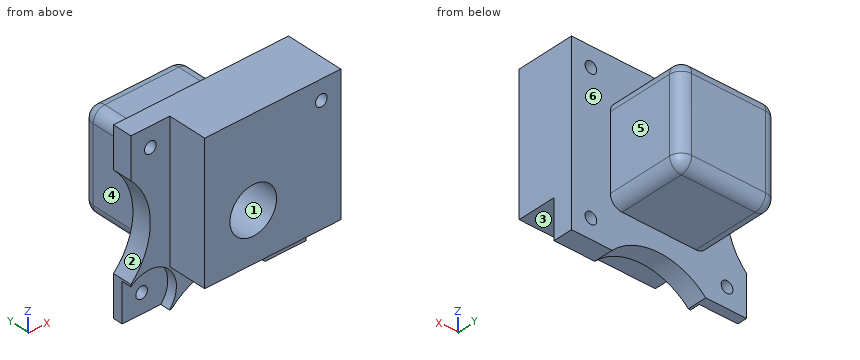
from build123d import *

# Parameters (mm, degrees)
SKETCH1_W               = 45
SKETCH1_H               = 45
BOSS_EXTRUDE1_DEPTH     = 15
CUT_EXTRUDE1_DEPTH      = 10
CUT_EXTRUDE2_DEPTH      = 38.243644172
CUT_EXTRUDE2_DEPTH_BACK = 38.243644172
CUT_EXTRUDE3_DEPTH      = 2.5
SKETCH5_W               = 25
SKETCH5_H               = 25
BOSS_EXTRUDE2_DEPTH     = 20
FILLET1_R               = 3
SKETCH6_R               = 6
CUT_EXTRUDE4_DEPTH      = 28.99918
SKETCH7_W               = 13
SKETCH7_H               = 13
CUT_EXTRUDE5_DEPTH      = 13
FILLET2_R               = 3
CUT_EXTRUDE6_DEPTH      = 42.074189356
CUT_EXTRUDE6_DEPTH_BACK = 42.074189356
SKETCH8_R               = 1.5


with BuildPart() as part:
    # Sketch1 → Boss-Extrude1 (new body)
    with BuildSketch(Plane(origin=(0, 0, 0), x_dir=(1, 0, 0), z_dir=(0, 1, 0))):
        with Locations((0.699698795, 4.865361446)):
            Rectangle(SKETCH1_W, SKETCH1_H)
    extrude(amount=BOSS_EXTRUDE1_DEPTH)

    # Sketch2 → Cut-Extrude1 (cut)
    with BuildSketch(Plane.XZ):
        Polygon((-21.800301205, 17.634638554), (-11.800301205, 17.634638554), (-11.800301205, -17.365361446), (23.199698795, -17.365361446), (23.199698795, -27.365361446), (-21.800301205, -27.365361446), align=None)
    extrude(amount=-CUT_EXTRUDE1_DEPTH, mode=Mode.SUBTRACT)

    # Sketch3 → Cut-Extrude2 (cut, two sides: drawn at the far end of the back side and taken through both)
    with BuildSketch(Plane.XZ.offset(-10).offset(-CUT_EXTRUDE2_DEPTH_BACK)):
        with BuildLine():
            Line((-11.340301205, -27.365361446), (12.739698795, -27.365361446))
            ThreePointArc((12.739698795, -27.365361446), (0.699698795, -22.366961339), (-11.340301205, -27.365361446))
        make_face()
        with BuildLine():
            Line((-21.800301205, 7.174638554), (-21.800301205, -16.905361446))
            ThreePointArc((-21.800301205, -16.905361446), (-16.801901098, -4.865361446), (-21.800301205, 7.174638554))
        make_face()
    extrude(amount=CUT_EXTRUDE2_DEPTH + CUT_EXTRUDE2_DEPTH_BACK, mode=Mode.SUBTRACT)

    # Sketch4 → Cut-Extrude3 (cut)
    with BuildSketch(Plane.XZ.offset(-10)):
        with BuildLine():
            Line((-21.800301205, -17.465361446), (-21.800301205, -27.365361446))
            Line((-21.800301205, -27.365361446), (-11.900301205, -27.365361446))
            ThreePointArc((-11.900301205, -27.365361446), (-12.153386497, -17.718446738), (-21.800301205, -17.465361446))
        make_face()
    extrude(amount=-CUT_EXTRUDE3_DEPTH, mode=Mode.SUBTRACT)

    # Sketch5 → Boss-Extrude2 (add)
    with BuildSketch(Plane(origin=(0, 15, 0), x_dir=(1, 0, 0), z_dir=(0, 1, 0))):
        with Locations((0.699698795, 4.865361446)):
            Rectangle(SKETCH5_W, SKETCH5_H)
    extrude(amount=BOSS_EXTRUDE2_DEPTH)

    # Fillet1
    fillet1_edges = [part.edges().sort_by_distance(p)[0] for p in [
        (-11.800301205, 25, -17.365361446),
        (-11.800301205, 25, 7.634638554),
        (13.199698795, 25, 7.634638554),
        (13.199698795, 25, -17.365361446),
        (-11.800301205, 35, -4.865361446),
        (0.699698795, 35, 7.634638554),
        (13.199698795, 35, -4.865361446),
        (0.699698795, 35, -17.365361446),
    ]]
    fillet(fillet1_edges, radius=FILLET1_R)

    # Sketch6 → Cut-Extrude4 (cut)
    with BuildSketch(Plane(origin=(0, 0, 0), x_dir=(-1, 0, 0), z_dir=(0, -1, 0))):
        with Locations(Location((-0.699698795, 4.865361446, 0), (0, 0, 90))):
            Circle(SKETCH6_R)
    extrude(amount=-CUT_EXTRUDE4_DEPTH, mode=Mode.SUBTRACT)

    # Sketch7 → Cut-Extrude5 (cut)
    with BuildSketch(Plane.XZ.offset(-28.99918)):
        with Locations((0.699698795, -4.865361446)):
            Rectangle(SKETCH7_W, SKETCH7_H)
    extrude(amount=CUT_EXTRUDE5_DEPTH, mode=Mode.SUBTRACT)

    # Fillet2
    fillet2_edges = [part.edges().sort_by_distance(p)[0] for p in [
        (-5.800301205, 28.99918, -4.865361446),
        (-5.800301205, 22.49918, 1.634638554),
        (0.699698795, 28.99918, -11.365361446),
        (-5.800301205, 22.49918, -11.365361446),
        (7.199698795, 28.99918, -4.865361446),
        (7.199698795, 22.49918, -11.365361446),
        (0.699698795, 28.99918, 1.634638554),
        (7.199698795, 22.49918, 1.634638554),
    ]]
    fillet(fillet2_edges, radius=FILLET2_R)

    # Sketch8 → Cut-Extrude6 (cut, two sides: drawn at the far end of the back side and taken through both)
    with BuildSketch(Plane(origin=(0, 15, 0), x_dir=(1, 0, 0), z_dir=(0, 1, 0)).offset(-CUT_EXTRUDE6_DEPTH_BACK)):
        with Locations(Location((-16.800301205, 22.365361446, 0), (0, 0, 270))):
            Circle(SKETCH8_R)
        with Locations(Location((18.199698795, 22.365361446, 0), (0, 0, 270))):
            Circle(SKETCH8_R)
        with Locations(Location((18.199698795, -12.634638554, 0), (0, 0, 270))):
            Circle(SKETCH8_R)
        with Locations(Location((-16.800301205, -12.634638554, 0), (0, 0, 270))):
            Circle(SKETCH8_R)
    extrude(amount=CUT_EXTRUDE6_DEPTH + CUT_EXTRUDE6_DEPTH_BACK, mode=Mode.SUBTRACT)


solid = part.part
Design review of the part built by this model. Coordinates are the model's own, in mm. Face numbers are marked on the shaded views. A direction names the side the tool comes from. Coordinates: 2 decimals unless noted, no trailing zeros. Loops run counter-clockwise (first coordinate to the right, second up) from the corner with the lowest first, then second, coordinate; pieces in that order, holes last. Notation, with made-up numbers: M 36,21.25 L 55,21.25 A20 ccw 55,58.25 Z; hole C 43,-39 d7. An arc over 180 degrees is marked long. Use one line per item in the form item = value.
(1) Consider section A-A (y = 17.5). Write out the cut boundary in (x, z), and give its area (3 significant figures).
Return value:
outline = M -11.8,-14.37 A3 ccw -8.8,-17.37 L 10.2,-17.37 A3 ccw 13.2,-14.37 L 13.2,4.63 A3 ccw 10.2,7.63 L -8.8,7.63 A3 ccw -11.8,4.63 Z; hole M -5.8,-8.37 A3 ccw -2.8,-11.37 L 4.2,-11.37 A3 ccw 7.2,-8.37 L 7.2,-1.37 A3 ccw 4.2,1.63 L -2.8,1.63 A3 ccw -5.8,-1.37 Z
area = 456 mm2
(2) Consider section B-B (z = 8.5). Write out the cut boundary in (x, y), and give its area (3 significant figures).
Return value:
outline = M -21.8,10 L -11.8,10 L -11.8,0 L 23.2,0 L 23.2,15 L -21.8,15 Z
area = 575 mm2
(3) Consider section C-C (x = -19). Write out the cut boundary in (y, z).
Return value:
outline = M 10,-15.92 L 12.5,-15.92 L 12.5,-27.37 L 15,-27.37 L 15,-13.23 L 10,-13.23 Z; M 10,3.5 L 15,3.5 L 15,17.63 L 10,17.63 Z
(4) Draft analysis for pull direction X (two halves, no side actions). For the marked faces 1, 2 and 3, state which applies: pulls with the +X half, pulls with the -X half, needs draft (parallel to the pull), parting line crosses it, or undercut.
Return value:
face_1 = undercut
face_2 = pulls with the -X half
face_3 = needs draft
(5) For the marked faces 4, 5 and 6, list the 3-axis set-ups (+Z, -Z, +X, -X, +Y, -Y) from which the entire face can be reached by the end or side of a thin tool; tool diameter is ignored.
Return value:
face_4 = +Z, -Z, -X, +Y
face_5 = +Z, -Z, +X, +Y
face_6 = +Y
(6) Clearance check with flat-ended pins moving along their axes: P1, Ø5, axis at x = -16.8, z = -22.37, coming from the +Y side; P2, Ø5.5, axis at x = 1.5, y = 20.5, coming from the +Z side; P3, Ø10, axis at y = 26.5, z = -4, coming from the -X side. State where each tip first meets the part, or that it passes through.
Return value:
P1 = 15
P2 = 7.63
P3 = -11.8
(7) For line 1 along X through (y, z) = (11, 12); line 2 along X through (y, z) = (4.5, 0); line 3 along Z through (x, y) = (17, 12.5), list the stretches that pass through material, from the lowest coordinate up. Write a range as from..to.
Return value:
line_1 = -21.8..-18.16, -15.44..16.84, 19.56..23.2
line_2 = -11.8..-2.81, 4.21..23.2
line_3 = -27.37..-23.27, -21.46..11.73, 13.54..17.63
(8) Consider section D-D (y = 13.5). Write out the cut boundary in (x, z), and give its area (3 significant figures).
Return value:
outline = M -21.8,-27.37 L -11.34,-27.37 A17 cw 12.74,-27.37 L 23.2,-27.37 L 23.2,17.63 L -21.8,17.63 L -21.8,7.17 A17 cw -21.8,-16.91 Z; hole C -16.8,-22.37 d3; hole C -16.8,12.63 d3; hole C 0.7,-4.87 d12; hole C 18.2,-22.37 d3; hole C 18.2,12.63 d3
area = 1,720 mm2
